Design review of the part built by this model. Coordinates are the model's own, in mm. Face numbers are marked on the shaded views. Give positions to 0.01 mm unless a question says otherwise; leave off trailing zeros. Write each loop counter-clockwise with the first axis right and the second up, starting at its lowest first coordinate (ties: lowest second). Pieces come first, ordered by that corner, then holes.
```python
from build123d import *
from build123d.topology import SkipClean

# Parameters (mm, degrees)
BOSS_EXTRUDE1_DEPTH     = 9.525
CUT_EXTRUDE4_DEPTH      = 4.7752
F_1_4_20_TAPPED_HOLE1_D = 5.1054


with BuildPart() as part:
    # Sketch1 → Boss-Extrude1 (new body)
    with BuildSketch(Plane.XY):
        with BuildLine():
            ThreePointArc((-22.767324083, 59.210121486), (-61.545192335, 15.374616506), (-47.937560329, -41.547320514))
            Line((-47.937560329, -41.547320514), (48.13808, -152.4))
            Line((48.13808, -152.4), (295.78808, -152.4))
            Line((295.78808, -152.4), (295.78808, 152.4))
            Line((295.78808, 152.4), (219.58808, 152.4))
            Line((219.58808, 152.4), (-22.767324083, 59.210121486))
        make_face()
    extrude(amount=-BOSS_EXTRUDE1_DEPTH)

    # Sketch1_5 → Cut-Extrude4 (cut)
    with SkipClean():  # keep this step's faces unmerged: merging them makes the solid invalid here
        with BuildSketch(Plane.XY):
            with BuildLine():
                Line((114.391061614, 111.949912244), (-22.767324083, 59.210121486))
                ThreePointArc((-22.767324083, 59.210121486), (35.915944774, 52.289907661), (63.4365, 0))
                ThreePointArc((63.4365, 0), (22.172037417, -59.435597827), (-47.937560329, -41.547320514))
                Line((-47.937560329, -41.547320514), (48.13808, -152.4))
                Line((48.13808, -152.4), (114.391061614, 111.949912244))
            make_face()
        extrude(amount=-CUT_EXTRUDE4_DEPTH, mode=Mode.SUBTRACT)

    # 1_4-20 Tapped Hole1 (through all)
    with Locations(Plane.XY):
        with Locations((283.08808, 127), (283.08808, -127), (130.68808, -127), (46.933080252, 19.440318364), (19.440318364, -46.933080252), (-46.933080252, -19.440318364), (-19.440318364, 46.933080252), (0, 0)):
            Hole(F_1_4_20_TAPPED_HOLE1_D / 2)


solid = part.part
```
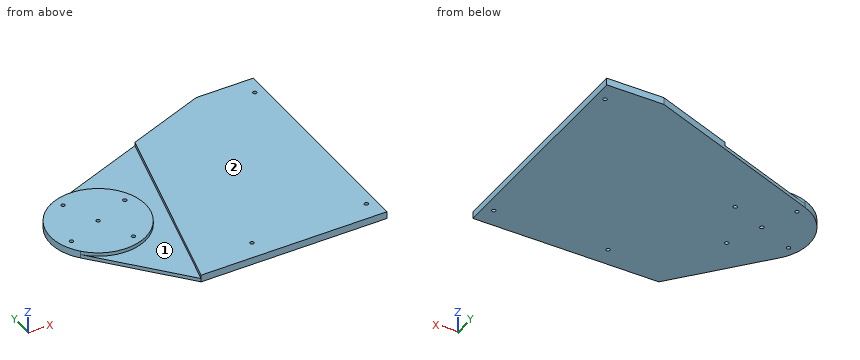
(1) Mouldability with a two-part tool opening along X and no side actions: class the marked faces 1 and 2 as pulls with the +X half, pulls with the -X half, needs draft (parallel to the pull), parting line crosses it, or undercut.
Resolved:
face 1: undercut
face 2: needs draft
(2) Consider section D-D, the plane y = -71. Give the boundary of the cut face in (x, z) (3 decimals), then the cut area to 3 significant figures.
Resolved:
outline: (-22.411, -9.525) - (295.788, -9.525) - (295.788, 0) - (68.539, 0) - (68.539, -4.775) - (-22.411, -4.775) - close
area: 2,600 mm2
(3) To check wall thickness, follow L1, parallel to Z at x = 38.5, y = 72.5 (3 decimals); L2, parallel to Y at x = 20.5, z = -9; L3, parallel to Y at x = 19, z = -1.25. State the ranges of each line that lie inside material, in increasing order.
Resolved:
L1: z = -9.525 to -4.775
L2: y = -120.51 to -49.26, -44.61 to 75.85
L3: y = -60.52 to -49.45, -44.42 to 60.52
(4) Clearance check with flat-ended pins moving along their axes: P1, Ø4, axis at y = -107.5, z = -8.5, coming from the -X side; P2, Ø3, axis at x = 130.69, y = -127, coming from the -Z side (3 decimals); P3, Ø3, axis at x = -10.5, z = -8.5, coming from the -Y side; P4, Ø4, axis at x = 33, z = -6, coming from the -Y side. State where each tip first meets the part, or that it passes through.
Resolved:
P1: stops at x = 7.49
P2: passes through
P3: stops at y = -86.47
P4: stops at y = -137.24
(5) Consider section B-B, the plane y = -10.5. Give the boundary of the cut face in (x, z) (3 decimals), then the cut area to 3 significant figures.
Resolved:
outline: (-62.561, -9.525) - (295.788, -9.525) - (295.788, 0) - (83.702, 0) - (83.702, -4.775) - (62.561, -4.775) - (62.561, 0) - (-62.561, 0) - close
area: 3,310 mm2
(6) Consider section A-A, the plane z = -2.25. Give the number of separate pieces and of enclosed holes in the cut face, then the cut area to 3 significant figures.
Resolved:
separate pieces: 2
enclosed holes: 8
area: 74,400 mm2
(7) Consider section C-C, the plane x = 77.5. Give the boundary of the cut face in (y, z) (3 decimals), then the cut area to 3 significant figures.
Resolved:
outline: (-152.4, -9.525) - (97.765, -9.525) - (97.765, -4.775) - (-35.246, -4.775) - (-35.246, 0) - (-152.4, 0) - close
area: 1,750 mm2
